Autodesk Inventor part; units mm, degrees
ref_plane "Work Plane1" through (1.525, 0, 0) normal (0, 0, 1) x (1, 0, 0)
ref_plane "YZ Plane" through (0, 0, 0) normal (1, 0, 0) x (0, 1, 0)
ref_plane "XZ Plane" through (0, 0, 0) normal (0, 1, 0) x (-1, 0, 0)
sketch "Sketch1" plane through (0, 0, 0) normal (0, 0, 1) x (1, 0, 0)
  line L0 (0, 2.94) -> (0, 2)
  line L1 (2.1, 2) -> (12, 2)
  line L2 (12, 2) -> (12, 0)
  line L3 (12, 0) -> (-0.4001, 0)
  line L4 (-2.8801, 0) -> (14.48, 0)
  line L5 (-0.4001, 0) -> (-0.4001, 2.94)
  line L6 (-0.4001, 2.94) -> (0, 2.94)
  line L7 (2.1, 2) -> (1.6705, 2)
  line L8 (1.6705, 2) -> (0, 2)
  line L9 (0, -0.588) -> (0, 3.528)
  dimension "d0" = 12
  dimension "d1" = 9.9
  dimension "d2" = 4
  dimension "d9" = 0.4001
  dimension "d10" = 5.88
  dimension "d13" = 0.4295
  dimension "d14" = 4
revolve "Body" add sketch "Sketch1" angle 360 about axis through (12, 0, 0) along (-1, 0, 0)
sketch "Sketch2" plane through (-0.4001, 0, 0) normal (-1, 0, 0) x (0, 0, 1)
  line L0 (0, 4.0415) -> (3.5, 2.0207)
  line L1 (3.5, 2.0207) -> (3.5, -2.0207)
  line L2 (3.5, -2.0207) -> (0, -4.0415)
  line L3 (0, -4.0415) -> (-3.5, -2.0207)
  line L4 (-3.5, -2.0207) -> (-3.5, 2.0207)
  line L5 (-3.5, 2.0207) -> (0, 4.0415)
  point P0 (0, 0)
  point P1 (0, 0)
  dimension "d11" = 7
extrude "Head" add sketch "Sketch2" along normal blind 2.4
sketch "Sketch4" plane through (0, 0, 0) normal (0, 0, 1) x (1, 0, 0)
  line L0 (-2.8001, 3.5) -> (-2.8001, 4.0415)
  line L1 (-2.8001, 4.0415) -> (-2.4875, 4.0415)
  line L2 (-2.4875, 4.0415) -> (-2.8001, 3.5)
  line L3 (-3.2801, 0) -> (0.0799, 0)
  line L4 (-0.4001, 4.0415) -> (-2.8001, 4.0415)
  line L5 (-2.8001, 2.0207) -> (-2.8001, 4.0415)
  dimension "d5" = 30
  dimension "d19" = 7
revolve "Chamfer1" cut sketch "Sketch4" angle 360 about axis through (-10, 0, 0) along (1, 0, 0)
thread "Thread"
chamfer "Chamfer2" distance 0.4294 distance2 0.4295 1 edges at (12, -2, 0) measured on face at (12, 0.1822, 0.4036)
ref_plane "Work Plane1" through (1.525, 0, 0) normal (0, 0, 1) x (1, 0, 0)
equation "\"d0\" = NLG"
equation "\"d1\" = GEL"
equation "\"d2\" = GD"
equation "\"d10\" = SD2"
equation "\"d14\" = BDM"
equation "\"d11\" = SW"
equation "\"d3\" = KOH - SD"
equation "\"d5\" = ANG1"
equation "\"d19\" = SW0"
equation "\"d15\" = GEL"
equation "\"d6\" = -0.5 * SPD + 0.5 * GD"
equation "\"NLG\" = 12"
equation "\"GD\" = NND"
equation "\"BDM\" = NND"
equation "\"KOH\" = 2.8"
equation "\"GEL\" = 9.9"
equation "\"SW\" = 7"
equation "\"SW0\" = SW"
equation "\"SPD\" = NND - 1.2269 * PTC"
equation "\"SD2\" = 5.88"
equation "\"SD\" = 0.4"
equation "\"ANG1\" = 30deg"
equation "\"GAL\" = 0.61345 * PTC"
equation "\"GUL\" = 0.61345 * PTC"
equation "\"RR\" = 0.2"
equation "\"GD1\" = THREADDIA - 1.2269 * PTC"
equation "\"THREADDIA\" = 4"
equation "\"SDH\" = SD2"
equation "\"SDHG\" = 2.1"
equation "\"TOA\" = 30deg"
equation "\"PTC\" = 0.7"
equation "\"NND\" = 4"
equation "\"E0\" = 8.085"
properties part number "ISO 4017 - M4 x 12" material "Stainless Steel, 440C"
Verification items for the finished model (mm, model axes). A direction names the side the tool comes from. Round coordinates to 2 decimals unless told otherwise and drop trailing zeros. Loops run counter-clockwise (first coordinate to the right, second up) from the corner with the lowest first, then second, coordinate; pieces in that order, holes last. Notation, with made-up numbers: (51.25, 43) -> (107.25, 43) arc R13 ccw to (107.25, 53) -> close; hole circle Ø1 at (37.25, 71.5). An arc over 180 degrees is marked (long way). Answer as a JSON object with one key per item and string values.
Q1. Section check A-A (x = -1.25). Record the boundary of the cut face in (y, z).
Data:
{"outline": "(-4.04, 0) -> (-2.02, -3.5) -> (2.02, -3.5) -> (4.04, 0) -> (2.02, 3.5) -> (-2.02, 3.5) -> close"}
Q2. Section check B-B (x = 10.5). Record the boundary of the cut face in (y, z), then the cut area to 3 significant figures.
Data:
{"outline": "circle Ø4 at (0, 0)", "area": "12.6 mm2"}
Q3. Go/stop test with flat-tipped pins: P1, Ø4, axis at x = 7.5, y = 0.5, coming from the +Z side; P2, Ø1, axis at x = -1, z = 2.5, coming from the +Y side; P3, Ø2, axis at x = 7, y = -2.5, coming from the -Z side. Record where each tip stops, or that it passes through.
Data:
{"P1": "stops at z = 2", "P2": "stops at y = 2.89", "P3": "stops at z = -1.32"}
Q4. Scan lines: line 1 (X direction, y = -1, z = 3.25); line 2 (Z direction, x = 10.5, y = 0); line 3 (X direction, y = -1, z = -2.5). Record each from-to range of solid material in increasing order. Write a range as from..to.
Data:
{"line 1": "x = -2.8..-0.4", "line 2": "z = -2..2", "line 3": "x = -2.8..0"}
Q5. Access from +Z, -Z, +X, -X, +Y, -Y to the whole of each face (thin tool, end or side, straight path). Record for faces 1 (the conical face through (-2.724, 1.808, -3.15)), 2 (the cylindrical face through (-0.2, 2.8, 0.9)).
Data:
{"face 1": "-Z, -X, +Y", "face 2": "+X"}
